```python
from build123d import *

# Parameters (mm, degrees)
SKETCH1_R           = 18
BOSS_EXTRUDE1_DEPTH = 100
SKETCH2_R           = 25
SKETCH2_R_2         = 15
CUT_EXTRUDE2_DEPTH  = 10
SKETCH4_R           = 3
CUT_EXTRUDE3_DEPTH  = 100
SKETCH5_R           = 18
SKETCH5_R_2         = 17
CUT_EXTRUDE4_DEPTH  = 1


with BuildPart() as part:
    # Sketch1 → Boss-Extrude1 (new body)
    with BuildSketch(Plane.XY):
        Circle(SKETCH1_R)
    extrude(amount=BOSS_EXTRUDE1_DEPTH)

    # Sketch2 → Cut-Extrude2 (cut)
    with BuildSketch(Plane.XY.offset(100)):
        Circle(SKETCH2_R)
        Circle(SKETCH2_R_2, mode=Mode.SUBTRACT)
    extrude(amount=-CUT_EXTRUDE2_DEPTH, mode=Mode.SUBTRACT)

    # Sketch4 → Cut-Extrude3 (cut)
    with BuildSketch(Plane.XY.offset(100)):
        Circle(SKETCH4_R)
    extrude(amount=-CUT_EXTRUDE3_DEPTH, mode=Mode.SUBTRACT)

    # Sketch5 → Cut-Extrude4 (cut)
    with BuildSketch(Plane(origin=(0, 0, 65), x_dir=(-1, 0, 0), z_dir=(0, 0, -1))):
        Circle(SKETCH5_R)
        Circle(SKETCH5_R_2, mode=Mode.SUBTRACT)
    extrude(amount=-CUT_EXTRUDE4_DEPTH, mode=Mode.SUBTRACT)


solid = part.part
```
Could you check a few things on this model? Use its own coordinates, in mm. A direction names the side the tool comes from. Give positions to 0.01 mm unless a question says otherwise; leave off trailing zeros. Loops run counter-clockwise (first coordinate to the right, second up) from the corner with the lowest first, then second, coordinate; pieces in that order, holes last. Notation, with made-up numbers: (-24.75, 57) -> (3.25, 57) arc R18 ccw to (3.25, 76) -> close; hole circle Ø4 at (66.5, 64.25). An arc over 180 degrees is marked (long way). Put each result on its own line as item: value.
(1) Thinking about a two-plate mould opening in Z: for faces 4 (the face through (0, -4, 0)), 5 (the face through (-7, -16, 65)), 6 (the face through (-2.343, 17.847, 77.832)), which applies, pulls with the +Z half, pulls with the -Z half, needs draft (parallel to the pull), parting line crosses it, or undercut?
Computed:
face 4: pulls with the -Z half
face 5: undercut
face 6: needs draft
(2) For faces 1 (the face through (-14.985, 0.66, 95.07)), 2 (the face through (-7, -16, 66)), 3 (the face through (-2.343, 17.847, 32.045)), which set-ups out of +Z, -Z, +X, -X, +Y, -Y let a thin tool reach every point of the face, with its end or its side?
Computed:
face 1: +Z
face 2: none
face 3: +Z, -Z
(3) Please list where these lines run through material, in increasing order: probe 1 along Y at (x, z) = (0, 73.5); probe 2 along Z at (x, y) = (-14.5, -9); probe 3 along Z at (x, y) = (16, -3.5). Write a range as [from, to].
Computed:
probe 1: [-18, -3], [3, 18]
probe 2: [0, 65], [66, 90]
probe 3: [0, 90]
(4) Imagine slicing it at A-A on x = 0. Write out the boundary of the cut face in (y, z).
Computed:
outline: (-18, 0) -> (-3, 0) -> (-3, 100) -> (-15, 100) -> (-15, 90) -> (-18, 90) -> (-18, 66) -> (-17, 66) -> (-17, 65) -> (-18, 65) -> close; (3, 0) -> (18, 0) -> (18, 65) -> (17, 65) -> (17, 66) -> (18, 66) -> (18, 90) -> (15, 90) -> (15, 100) -> (3, 100) -> close
(5) I'm going to push flat-ended pins straight in: pin 1 Ø5 at (x, z) = (-13.5, 56) entering from +Y; pin 2 Ø8 at (y, z) = (14, 13) entering from -X; pin 3 Ø2 at (x, z) = (-7, 42.5) entering from -Y. Where does each tip first touch, or does it pass through?
Computed:
pin 1: y = 14.25
pin 2: x = -14.97
pin 3: y = -16.97
(6) Imagine slicing it at D-D on y = -7. Write out the boundary of the cut face in (x, z), plus the area to 3 significant figures.
Computed:
outline: (-16.58, 0) -> (16.58, 0) -> (16.58, 65) -> (15.49, 65) -> (15.49, 66) -> (16.58, 66) -> (16.58, 90) -> (13.27, 90) -> (13.27, 100) -> (-13.27, 100) -> (-13.27, 90) -> (-16.58, 90) -> (-16.58, 66) -> (-15.49, 66) -> (-15.49, 65) -> (-16.58, 65) -> close
area: 3,250 mm^2
(7) Imagine slicing it at C-C on z = 81.5. Write out the boundary of the cut face in (x, y).
Computed:
outline: circle Ø36 at (0, 0); hole circle Ø6 at (0, 0)
